Could you check a few things on this drawing? It's one solid part, dimensions in mm from its lowest x, y, z. A direction names the side the tool comes from. Give positions to 0.01 mm unless a question says otherwise; leave off trailing zeros. Order: outer loops, then holes, each group sorted by start corner. A loop starts at its lowest first (then second) coordinate and runs counter-clockwise, first axis right, second up. Notation, with made-up numbers: (35, 75.25) -> (50, 75.25) arc R9 cw to (50, 83.25) -> close; hole circle Ø4 at (-36, -22). An arc over 180 degrees is marked (long way). Answer as CSV lines item,"result".
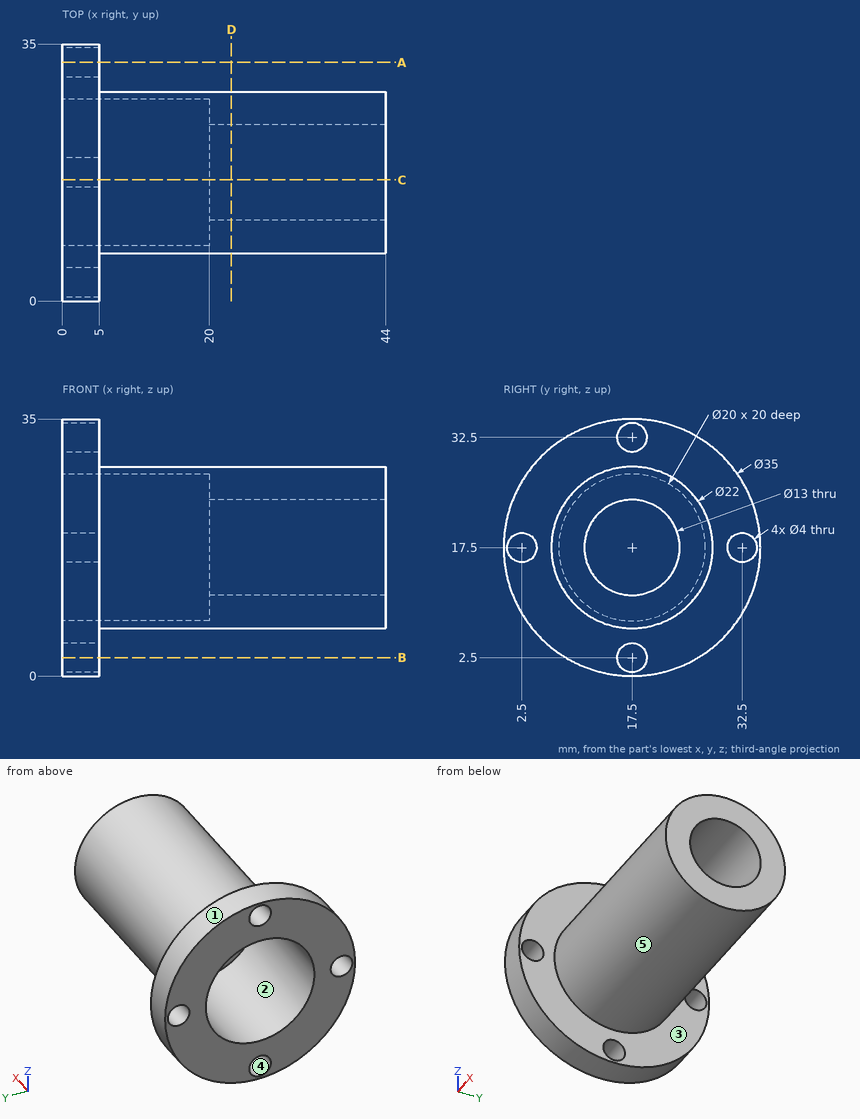
Item 1: Please list where these lines run through material, in increasing order: line 1 along Z through (x, y) = (35.75, 17.5); line 2 along Y through (x, z) = (1, 17); line 3 along Z through (x, y) = (7.25, 17.5).
Numbers:
line 1,"z = 6.5 to 11, 24 to 28.5"
line 2,"y = 0.01 to 0.56, 4.44 to 7.51, 27.49 to 30.56, 34.44 to 34.99"
line 3,"z = 6.5 to 7.5, 27.5 to 28.5"
Item 2: Imagine slicing it at C-C, the plane y = 16.5. Please give me the cut outline in (x, z), then the cut area to 3 significant figures.
Numbers:
outline,"(0, 0.03) -> (5, 0.03) -> (5, 0.77) -> (0, 0.77) -> close; (0, 4.23) -> (5, 4.23) -> (5, 6.55) -> (44, 6.55) -> (44, 11.08) -> (20, 11.08) -> (20, 7.55) -> (0, 7.55) -> close; (0, 27.45) -> (20, 27.45) -> (20, 23.92) -> (44, 23.92) -> (44, 28.45) -> (5, 28.45) -> (5, 30.77) -> (0, 30.77) -> close; (0, 34.23) -> (5, 34.23) -> (5, 34.97) -> (0, 34.97) -> close"
area,"288 mm²"
Item 3: Imagine slicing it at A-A, the plane y = 32.5. Please give me the cut outline in (x, z).
Numbers:
outline,"(0, 8.49) -> (5, 8.49) -> (5, 15.5) -> (0, 15.5) -> close; (0, 19.5) -> (5, 19.5) -> (5, 26.51) -> (0, 26.51) -> close"
Item 4: For pin 1 (2 mm diameter, centred on x = 22, y = 16.5, fed in from -Z); pin 2 (6.5 mm diameter, centred on y = 17.5, z = 2.5, fed in from +X); pin 3 (5 mm diameter, centred on x = 32, y = 12.5, fed in from -Z), each with a flat end and sliding along its axis, tell me the tip position at first contact or that it passes through.
Numbers:
pin 1,"stops at z = 6.5"
pin 2,"stops at x = 5"
pin 3,"stops at z = 6.79"
Item 5: Imagine slicing it at D-D, the plane x = 23. Please give me the cut outline in (y, z).
Numbers:
outline,"circle Ø22 at (17.5, 17.5); hole circle Ø13 at (17.5, 17.5)"
Item 6: We'd pull the mould along Y, two halves only. Please class the marked faces 1, 2 and 3: released by +Y, released by -Y, zero draft, split by the parting line, or undercut.
Numbers:
face 1,"split by the parting line"
face 2,"undercut"
face 3,"zero draft"
Item 7: For the marked faces 4 and 5, which set-ups out of +Z, -Z, +X, -X, +Y, -Y let a thin tool reach every point of the face, with its end or its side?
Numbers:
face 4,"+X, -X"
face 5,"+X"
